Can you work these out from the model? Positions are in its coordinate system, mm. A direction names the side the tool comes from. Coordinates: 2 decimals unless noted, no trailing zeros. Order: outer loops, then holes, each group sorted by start corner. A loop starts at its lowest first (then second) coordinate and runs counter-clockwise, first axis right, second up. Notation, with made-up numbers: (-39, -32) -> (-17, -32) arc R30 ccw to (-17, 5) -> close; hole circle Ø5 at (80.5, -36). An arc over 180 degrees is marked (long way). Answer in a Markdown table with one row per item.
```python
from build123d import *

# Parameters (mm, degrees)
F0_W     = 12.7
F0_H     = 1.6002
F0_H_2   = 1.5494
F0_W_2   = 1.6002
F1_DEPTH = 3.175
F2_T     = -1.6002
F3_DEPTH = 25.4
F4_W     = 12.7
F4_H     = 1.6002
F4_W_2   = 1.6002
F4_H_2   = 1.5494
F5_DEPTH = 1.6002


with BuildPart() as f1:
    # F0 (on Top) → F1 (new body)
    with BuildSketch(Plane.XY):
        with Locations((-5.0789434463, 30.2115620618)):
            Rectangle(F0_W, F0_H)
        with Locations((-5.0789434463, 28.6113620618)):
            Rectangle(F0_W, F0_H)
        with Locations((-5.0789434463, 25.4363620618)):
            Rectangle(F0_W, F0_H_2)
        with Locations((-5.0789434463, 23.8615620618)):
            Rectangle(F0_W, F0_H)
        with Locations((-5.0789434463, 27.0111620618)):
            Rectangle(F0_W, F0_H)
        with Locations((-12.2290434463, 30.2115620618)):
            Rectangle(F0_W_2, F0_H)
        with Locations((-12.2290434463, 27.0111620618)):
            Rectangle(F0_W_2, F0_H)
        with Locations((-12.2290434463, 23.8615620618)):
            Rectangle(F0_W_2, F0_H)
        with Locations((2.0711565537, 30.2115620618)):
            Rectangle(F0_W_2, F0_H)
        with Locations((2.0711565537, 27.0111620618)):
            Rectangle(F0_W_2, F0_H)
        with Locations((2.0711565537, 23.8615620618)):
            Rectangle(F0_W_2, F0_H)
        with Locations((-12.2290434463, 28.6113620618)):
            Rectangle(F0_W_2, F0_H)
        with Locations((-12.2290434463, 25.4363620618)):
            Rectangle(F0_W_2, F0_H_2)
        with Locations((2.0711565537, 28.6113620618)):
            Rectangle(F0_W_2, F0_H)
        with Locations((2.0711565537, 25.4363620618)):
            Rectangle(F0_W_2, F0_H_2)
    extrude(amount=F1_DEPTH)

    # F2
    f2_openings = [f1.faces().sort_by_distance(p)[0] for p in [
        (-5.078943, 27.036562, 0),
    ]]
    offset(amount=F2_T, openings=f2_openings)

    # F0 (on Top) → F3 (cut)
    with BuildSketch(Plane.XY):
        with Locations((-5.0789434463, 25.4363620618)):
            Rectangle(F0_W, F0_H_2)
        with Locations((-5.0789434463, 28.6113620618)):
            Rectangle(F0_W, F0_H)
    extrude(amount=F3_DEPTH, mode=Mode.SUBTRACT)

    # F4 (on face) → F5 (cut)
    with BuildSketch(Plane.XY.offset(3.175)):
        with Locations((-5.0789434463, 28.6113620618)):
            Rectangle(F4_W, F4_H)
        with Locations((2.0711565537, 28.6113620618)):
            Rectangle(F4_W_2, F4_H)
        with Locations((-12.2290434463, 28.6113620618)):
            Rectangle(F4_W_2, F4_H)
        with Locations((2.0711565537, 25.4363620618)):
            Rectangle(F4_W_2, F4_H_2)
        with Locations((-12.2290434463, 25.4363620618)):
            Rectangle(F4_W_2, F4_H_2)
    extrude(amount=-F5_DEPTH, mode=Mode.SUBTRACT)


solid = f1.part
```
(1) On a 3-axis mill with a long thin cutter (end or side, diameter ignored), from which of +Z, -Z, +X, -X, +Y, -Y can I reach the whole of each face in a straight line? I mean faces 4 (the flat face through (-5, 24.662, 2)), 5 (the flat face through (-5, 24, 0)), 6 (the flat face through (-5, 24, 3.175)), 7 (the flat face through (-5, 26.211, 2)), 8 (the flat face through (1.271, 27, 1)). Say none if no direction works.
Response values:
| item | result |
|---|---|
| face 4 | +Z |
| face 5 | -Z, +X, -X, +Y, -Y |
| face 6 | +Z, +X, -X, +Y, -Y |
| face 7 | +Z, +X, -X |
| face 8 | -Z |
(2) Suppose I cut it at D-D (y = 26.75). Please give me the cut outline in (x, z) (3 decimals), and give its area (3 significant figures).
Response values:
| item | result |
|---|---|
| outline | (-13.029, 0) -> (-11.429, 0) -> (-11.429, 1.575) -> (1.271, 1.575) -> (1.271, 0) -> (2.871, 0) -> (2.871, 3.175) -> (-13.029, 3.175) -> close |
| area | 30.5 mm2 |
(3) Will these pins go through, and if not, where does the flat tip stop? pin 1 Ø1.3 at (x, y) = (2, 28.5) entering from +Z; pin 2 Ø0.8 at (x, y) = (-5, 27) entering from -Z.
Response values:
| item | result |
|---|---|
| pin 1 | z = 1.57 |
| pin 2 | z = 1.57 |
(4) Suppose I cut it at C-C (x = -2). Please give me the cut outline in (y, z) (3 decimals), and give its area (3 significant figures).
Response values:
| item | result |
|---|---|
| outline | (23.061, 0) -> (24.662, 0) -> (24.662, 3.175) -> (23.061, 3.175) -> close; (26.211, 1.575) -> (27.811, 1.575) -> (27.811, 3.175) -> (26.211, 3.175) -> close; (29.411, 0) -> (31.012, 0) -> (31.012, 3.175) -> (29.411, 3.175) -> close |
| area | 12.7 mm2 |
(5) I need wall thicknesses on line 1 (Y direction, x = -9.5, z = 2.3); line 2 (X direction, y = 28.5, z = 0.55); line 3 (Y direction, x = -4.75, z = 0.9). Which ranges of each line are inside material? Lowest first, please. Write a range as [from, to].
Response values:
| item | result |
|---|---|
| line 1 | [23.06, 24.66], [26.21, 27.81], [29.41, 31.01] |
| line 2 | [-13.03, -11.43], [1.27, 2.87] |
| line 3 | [23.06, 24.66], [29.41, 31.01] |
(6) We'd pull the mould along X, two halves only. Please class faces 1 (the flat face through (-5, 29.411, 2)), 2 (the flat face through (-13.029, 27, 1)), 3 (the flat face through (-5, 27.811, 2)): +X half, -X half, draft (parallel to the pull), parting line (faces both ways), or undercut.
Response values:
| item | result |
|---|---|
| face 1 | undercut |
| face 2 | -X half |
| face 3 | draft |
(7) Suppose I cut it at A-A (z = 2). Please give me the cut outline in (x, y).
Response values:
| item | result |
|---|---|
| outline | (-13.03, 23.06) -> (2.87, 23.06) -> (2.87, 24.66) -> (-13.03, 24.66) -> close; (-13.03, 26.21) -> (2.87, 26.21) -> (2.87, 27.81) -> (-13.03, 27.81) -> close; (-13.03, 29.41) -> (2.87, 29.41) -> (2.87, 31.01) -> (-13.03, 31.01) -> close |
(8) Suppose I cut it at B-B (y = 25). Please give me the cut outline in (x, z), and give its area (3 significant figures).
Response values:
| item | result |
|---|---|
| outline | (-13.03, 0) -> (-11.43, 0) -> (-11.43, 1.57) -> (-13.03, 1.57) -> close; (1.27, 0) -> (2.87, 0) -> (2.87, 1.57) -> (1.27, 1.57) -> close |
| area | 5.04 mm2 |
